Geometry check sheet. Reference: the model listing, model coordinates, mm. A direction names the side the tool comes from. Round coordinates to 2 decimals unless told otherwise and drop trailing zeros. Order: outer loops, then holes, each group sorted by start corner. A loop starts at its lowest first (then second) coordinate and runs counter-clockwise, first axis right, second up. Notation, with made-up numbers: (27.25, -1.5) - (35.25, -1.5) arc R24 cw to (35.25, 9.5) - close; hole circle Ø11 at (-29, 14.5). An arc over 180 degrees is marked (long way). Use a Markdown table: item, result. Add a question column.
(1) Mould release check, pull along X, two halves, no side actions. Record for faces 4 (the face through (-9, 1, 2.5)), 5 (the face through (-0.059, 7.563, 2.254)), 6 (the face through (9.121, 2.872, 1.845)): released by +X, released by -X, zero draft, split by the parting line, or undercut.
(2) Thickness scan on line 1 along Y through (x, z) = (0, -1.8); line 2 along Z through (x, y) = (-4.5, -3); line 3 along X through (y, z) = (-4.75, 2.25). Record the ranges inside material, lowest first. Write a range as [from, to].
(3) Section check A-A on x = 0. Record the boundary of the cut face in (y, z), then the cut area to 3 significant figures.
(4) Section check B-B on z = -1.8. Record the boundary of the cut face in (x, y), then the cut area to 3 significant figures.
(5) Access from +Z, -Z, +X, -X, +Y, -Y to the whole of each face (thin tool, end or side, straight path). Record for faces 1 (the face through (-2, -4, 0)), 2 (the face through (2, 0, 2)), 3 (the face through (0, 0, 2.5)).
(6) Section check C-C on z = 0.25. Record the boundary of the cut face in (x, y), then the cut area to 3 significant figures.
(7) Gauge pin test, flat ends, axial feed: P1, Ø1, axis at y = 5.5, z = 1.5, coming from the +X side; P2, Ø1.5, axis at x = 1.5, z = -2, coming from the +Y side; P3, Ø3, axis at x = 0, y = 0, coming from the -Z side. Record the tip position at first contact, or that the pin passes through.
```python
from build123d import *

# Parameters (mm, degrees)
F0_R     = 9.5631
F1_DEPTH = 2.5
F2_R     = 1.729466
F3_DEPTH = 0.5
F4_R     = 4
F5_DEPTH = 3.5
F6_R     = 1.207107
F7_R     = 2
F8_DEPTH = 3
F9_R     = 0.79669


with BuildPart() as f1:
    # F0 (on Top) → F1 (new body)
    with BuildSketch(Plane.XY):
        Circle(F0_R)
    extrude(amount=F1_DEPTH)

    # F2 (on face) → F3 (cut)
    with BuildSketch(Plane.XY.offset(2.5)):
        with BuildLine():
            ThreePointArc((-4.01538, 6.40915), (0, 7.5631), (4.01538, 6.40915))
            Line((4.01538, 6.40915), (4.515668, 7.275673))
            ThreePointArc((4.515668, 7.275673), (0, 8.5631), (-4.515668, 7.275673))
            Line((-4.515668, 7.275673), (-4.01538, 6.40915))
        make_face()
        with BuildLine():
            Line((4.515668, 7.275673), (4.01538, 6.40915))
            ThreePointArc((4.01538, 6.40915), (6.549837, 3.78155), (7.558177, 0.272846))
            Line((7.558177, 0.272846), (8.558752, 0.272846))
            ThreePointArc((8.558752, 0.272846), (7.415862, 4.28155), (4.515668, 7.275673))
        make_face()
        with BuildLine():
            ThreePointArc((-7.558177, 0.272846), (-6.549837, 3.78155), (-4.01538, 6.40915))
            Line((-4.01538, 6.40915), (-4.515668, 7.275673))
            ThreePointArc((-4.515668, 7.275673), (-7.415862, 4.28155), (-8.558752, 0.272846))
            Line((-8.558752, 0.272846), (-7.558177, 0.272846))
        make_face()
        with BuildLine():
            Line((8.558752, 0.272846), (7.558177, 0.272846))
            ThreePointArc((7.558177, 0.272846), (7.561869, 0.136445), (7.5631, 0))
            ThreePointArc((7.5631, 0), (6.480548, -3.8991), (3.542796, -6.681996))
            Line((3.542796, -6.681996), (4.043084, -7.54852))
            ThreePointArc((4.043084, -7.54852), (7.3467, -4.399167), (8.5631, 0))
            ThreePointArc((8.5631, 0), (8.562013, 0.136441), (8.558752, 0.272846))
        make_face()
        with BuildLine():
            ThreePointArc((-3.542796, -6.681996), (-6.549837, -3.78155), (-7.558177, 0.272846))
            Line((-7.558177, 0.272846), (-8.558752, 0.272846))
            ThreePointArc((-8.558752, 0.272846), (-7.415862, -4.28155), (-4.043084, -7.54852))
            Line((-4.043084, -7.54852), (-3.542796, -6.681996))
        make_face()
        with BuildLine():
            ThreePointArc((3.542796, -6.681996), (0, -7.5631), (-3.542796, -6.681996))
            Line((-3.542796, -6.681996), (-4.043084, -7.54852))
            ThreePointArc((-4.043084, -7.54852), (0, -8.5631), (4.043084, -7.54852))
            Line((4.043084, -7.54852), (3.542796, -6.681996))
        make_face()
        with BuildLine():
            Line((4.01538, 6.40915), (1.594189, 2.215524))
            ThreePointArc((1.594189, 2.215524), (0, 2.729466), (-1.594189, 2.215524))
            Line((-1.594189, 2.215524), (-4.01538, 6.40915))
            ThreePointArc((-4.01538, 6.40915), (-6.549837, 3.78155), (-7.558177, 0.272846))
            Line((-7.558177, 0.272846), (-2.715795, 0.272846))
            ThreePointArc((-2.715795, 0.272846), (-2.363787, -1.364733), (-1.121605, -2.48837))
            Line((-1.121605, -2.48837), (-3.542796, -6.681996))
            ThreePointArc((-3.542796, -6.681996), (0, -7.5631), (3.542796, -6.681996))
            Line((3.542796, -6.681996), (1.121605, -2.48837))
            ThreePointArc((1.121605, -2.48837), (2.363787, -1.364733), (2.715795, 0.272846))
            Line((2.715795, 0.272846), (7.558177, 0.272846))
            ThreePointArc((7.558177, 0.272846), (6.549837, 3.78155), (4.01538, 6.40915))
        make_face()
        Circle(F2_R, mode=Mode.SUBTRACT)
    extrude(amount=-F3_DEPTH, mode=Mode.SUBTRACT)

    # F4 (on face) → F5 (join)
    with BuildSketch(Plane(origin=(0, 0, 0), x_dir=(1, 0, 0), z_dir=(0, 0, -1))):
        Circle(F4_R)
    extrude(amount=F5_DEPTH)

    # F6
    f6_edges = [f1.edges().sort_by_distance(p)[0] for p in [
        (-9.5631, 0, 0),
    ]]
    fillet(f6_edges, radius=F6_R)

    # F7 (on face) → F8 (cut)
    with BuildSketch(Plane(origin=(0, 0, -3.5), x_dir=(1, 0, 0), z_dir=(0, 0, -1))):
        Circle(F7_R)
    extrude(amount=-F8_DEPTH, mode=Mode.SUBTRACT)

    # F9
    f9_edges = [f1.edges().sort_by_distance(p)[0] for p in [
        (-4, 0, -3.5),
    ]]
    fillet(f9_edges, radius=F9_R)


solid = f1.part
```
Check sheet entries:
| question | item | result |
|---|---|---|
| 1 | face 4 | zero draft |
| 1 | face 5 | undercut |
| 1 | face 6 | split by the parting line |
| 2 | line 1 | y = [-4, -2], [2, 4] |
| 2 | line 2 | z = [0, 2.5] |
| 2 | line 3 | x = [-8.3, -7.12], [-5.89, -2.43], [2.43, 5.89], [7.12, 8.3] |
| 3 | outline | (-9.56, 1.21) arc R1.21 ccw to (-8.36, 0) - (-4, 0) - (-4, -2.7) arc R0.8 ccw to (-3.2, -3.5) - (-2, -3.5) - (-2, -0.5) - (2, -0.5) - (2, -3.5) - (3.2, -3.5) arc R0.8 ccw to (4, -2.7) - (4, 0) - (8.36, 0) arc R1.21 ccw to (9.56, 1.21) - (9.56, 2.5) - (8.56, 2.5) - (8.56, 2) - (7.56, 2) - (7.56, 2.5) - (2.73, 2.5) - (2.73, 2) - (1.73, 2) - (1.73, 2.5) - (-1.73, 2.5) - (-1.73, 2) - (-8.56, 2) - (-8.56, 2.5) - (-9.56, 2.5) - close |
| 3 | area | 58.5 mm2 |
| 4 | outline | circle Ø8 at (0, 0); hole circle Ø4 at (0, 0) |
| 4 | area | 37.7 mm2 |
| 5 | face 1 | -Z |
| 5 | face 2 | +Z |
| 5 | face 3 | +Z, +X, -X, +Y, -Y |
| 6 | outline | circle Ø18.18 at (0, 0) |
| 6 | area | 260 mm2 |
| 7 | P1 | stops at x = 8.15 |
| 7 | P2 | stops at y = 3.93 |
| 7 | P3 | stops at z = -0.5 |
